Autodesk Inventor part; units mm, degrees
ref_plane "YZ Plane" through (0, 0, 0) normal (1, 0, 0) x (0, 1, 0)
ref_plane "XZ Plane" through (0, 0, 0) normal (0, 1, 0) x (-1, 0, 0)
ref_plane "XY Plane" through (0, 0, 0) normal (0, 0, 1) x (1, 0, 0)
sketch "Boceto1" plane through (0, 0, 0) normal (0, 1, 0) x (1, 0, 0)
  line L0 (-7.5, 5) -> (7.5, 5)
  line L1 (7.5, 5) -> (7.5, -5)
  line L2 (7.5, -5) -> (-7.5, -5)
  line L3 (-7.5, -5) -> (-7.5, 5)
  line L4 (-10.5, 0) -> (10.5, 0)
  line L5 (0, -7) -> (0, 7)
  dimension "d0" = 15
  dimension "d1" = 10
extrude "Extrusión1" add sketch "Boceto1" along normal blind 3
sketch "Boceto2" plane through (-7.5, 0, 5) normal (0, 0, 1) x (1, 0, 0)
  line L0 (15, 3) -> (0, 3)
  line L1 (0, 3) -> (0, 13)
  line L2 (0, 13) -> (15, 13)
  line L3 (15, 13) -> (15, 10)
  line L4 (15, 10) -> (3, 10)
  line L5 (3, 10) -> (3, 3)
  point P0 (7.5, 0)
  dimension "d5" = 10
  dimension "d6" = 3
  dimension "d7" = 15
  dimension "d8" = 12
extrude "Extrusión2" add sketch "Boceto2" against normal up to surface (10 mm away)
sketch "Boceto3" plane through (-7.5, 13, 5) normal (0, 1, 0) x (1, 0, 0)
  circle A0 centre (7.5, 5) radius 1.5
  dimension "d11" = 3
extrude "Extrusión3" cut sketch "Boceto3" against normal up to surface (3 mm away)
fillet "Empalme1" radius 2 2 edges at (-4.5, 10, 0) (-4.5, 3, 0)
sketch "Boceto4" plane through (0, 0, 0) normal (0, -1, 0) x (-1, 0, 0)
  circle A0 centre (0, 0) radius 2
  dimension "d15" = 4
extrude "Extrusión4" cut sketch "Boceto4" against normal up to surface (3 mm away)
fillet "Empalme2" radius 1 4 edges at (7.5, 0, 0) (7.5, 3, 0) (7.5, 13, 0) (7.5, 10, 0)
fillet "Empalme3" radius 4 2 edges at (-7.5, 13, 0) (-7.5, 0, 0)
fillet "Empalme4" radius 0.5 32 edges at (-6.3284, 1.1716, -5) (-7.5, 6.5, -5) (-6.3284, 11.8284, -5) (1.5, 13, -5) (7.2071, 12.7071, -5) (7.5, 11.5, -5) (7.2071, 10.2929, -5) (2, 10, -5) (-3.9142, 9.4142, -5) (-4.5, 6.5, -5) (-3.9142, 3.5858, -5) (2, 3, -5) (7.2071, 2.7071, -5) (7.5, 1.5, -5) (7.2071, 0.2929, -5) (1.5, 0, -5) (7.2071, 0.2929, 5) (7.5, 1.5, 5) (7.2071, 2.7071, 5) (2, 3, 5) (-3.9142, 3.5858, 5) (-4.5, 6.5, 5) (-3.9142, 9.4142, 5) (2, 10, 5) (7.2071, 10.2929, 5) (7.5, 11.5, 5) (7.2071, 12.7071, 5) (1.5, 13, 5) (-6.3284, 11.8284, 5) (-7.5, 6.5, 5) (-6.3284, 1.1716, 5) (1.5, 0, 5)
chamfer "Chaflán1" distance 1 angle 45 1 edges at (-1.5, 10, 0)
properties part number "Cable-Holder"
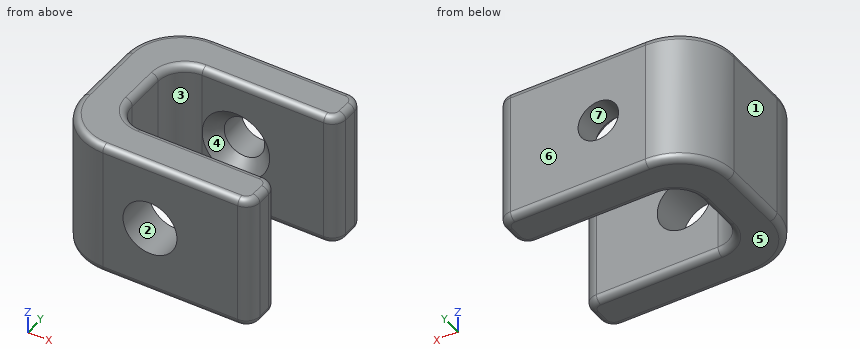
Source: CAD feature listing. Evaluate the final solid. Frame: model axes, mm. Face numbers are marked on the shaded views. A direction names the side the tool comes from. Coordinates: 2 decimals unless noted, no trailing zeros. Write each loop counter-clockwise with the first axis right and the second up, starting at its lowest first coordinate (ties: lowest second). Pieces come first, ordered by that corner, then holes. Notation, with made-up numbers: M -22,44 L 26,44 A18 cw 26,67 Z; hole C -5.5,36.25 d11. An arc over 180 degrees is marked long. Use a Markdown table: item, result.
1) First-contact query: pin 1 Ø3 at (y, z) = (6.5, -0.5) entering from +X; pin 2 Ø1.5 at (y, z) = (3.5, -3) entering from +X. Flat tips, straight axial feed; report the tip coordinate or a pass-through.
Conclusion:
| item | result |
|---|---|
| pin 1 | stops at x = -4.5 |
| pin 2 | stops at x = 7.16 |
2) Section D-D, the plane z = -4. Output: boundary loops of the cut face in (x, y), then the cut area to 3 significant figures.
Conclusion:
| item | result |
|---|---|
| outline | M -7.5,4 A4 ccw -3.5,0 L 6.5,0 A1 ccw 7.5,1 L 7.5,2 A1 ccw 6.5,3 L -2.5,3 A2 cw -4.5,5 L -4.5,8 A2 cw -2.5,10 L 6.5,10 A1 ccw 7.5,11 L 7.5,12 A1 ccw 6.5,13 L -3.5,13 A4 ccw -7.5,9 Z |
| area | 105 mm^2 |
3) Section A-A, the plane z = 0. Give the number of separate pieces and of enclosed holes in the cut face, then the cut area to 3 significant figures.
Conclusion:
| item | result |
|---|---|
| separate pieces | 3 |
| enclosed holes | 0 |
| area | 83.0 mm^2 |
4) Reachability of the marked faces 1, 2 and 3 from +Z, -Z, +X, -X, +Y, -Y: full face, straight path, thin tool, end or side. Return the list, or none.
Conclusion:
| item | result |
|---|---|
| face 1 | +Z, -Z, -X, +Y, -Y |
| face 2 | -Y |
| face 3 | +Z, -Z, +X |
5) Mould query, pull axis Z, two halves, no side actions, for the marked faces 4, 5, 6 and 7. Classes: pulls with the +Z half, pulls with the -Z half, needs draft (parallel to the pull), parting line crosses it, or undercut.
Conclusion:
| item | result |
|---|---|
| face 4 | undercut |
| face 5 | pulls with the -Z half |
| face 6 | needs draft |
| face 7 | undercut |
6) Ray query, L1, parallel to Y at x = 4.25, z = -0.5; L2, parallel to Z at x = 0, y = 11.95; L3, parallel to X at y = 5.75, z = -1.75. Return the intervals inside material, ascending.
Conclusion:
| item | result |
|---|---|
| L1 | y = 0 to 3, 10 to 13 |
| L2 | z = -5 to -1.5, 1.5 to 5 |
| L3 | x = -7.5 to -4.5 |
7) Section C-C, the plane x = 0. Output: boundary loops of the cut face in (y, z).
Conclusion:
| item | result |
|---|---|
| outline | M 0,-4.5 A0.5 ccw 0.5,-5 L 2.5,-5 A0.5 ccw 3,-4.5 L 3,-2 L 0,-2 Z; M 0,2 L 3,2 L 3,4.5 A0.5 ccw 2.5,5 L 0.5,5 A0.5 ccw 0,4.5 Z; M 10,-4.5 A0.5 ccw 10.5,-5 L 12.5,-5 A0.5 ccw 13,-4.5 L 13,-1.5 L 11,-1.5 L 10,-2.5 Z; M 10,2.5 L 11,1.5 L 13,1.5 L 13,4.5 A0.5 ccw 12.5,5 L 10.5,5 A0.5 ccw 10,4.5 Z |
8) Section B-B, the plane x = 2.75. Output: boundary loops of the cut face in (y, z), then the cut area to 3 significant figures.
Conclusion:
| item | result |
|---|---|
| outline | M 0,-4.5 A0.5 ccw 0.5,-5 L 2.5,-5 A0.5 ccw 3,-4.5 L 3,4.5 A0.5 ccw 2.5,5 L 0.5,5 A0.5 ccw 0,4.5 Z; M 10,-4.5 A0.5 ccw 10.5,-5 L 12.5,-5 A0.5 ccw 13,-4.5 L 13,4.5 A0.5 ccw 12.5,5 L 10.5,5 A0.5 ccw 10,4.5 Z |
| area | 59.6 mm^2 |
